Autodesk Fusion 360 part; units mm, degrees
sketch "Sketch1" plane through (0, 0, 0) normal (0, 0, 1) x (1, 0, 0)
  line L0 (-35.5, 22) -> (35.5, 22)
  line L1 (35.5, 22) -> (35.5, -22)
  line L2 (35.5, -22) -> (-35.5, -22)
  line L3 (-35.5, -22) -> (-35.5, 22)
  line L4 (0, 0) -> (-35.5, 0) construction
  line L5 (0, 0) -> (0, 22) construction
  circle A0 centre (-32.5, 19) radius 1.5
  circle A1 centre (32.5, 19) radius 1.5
  circle A2 centre (-32.5, -19) radius 1.5
  circle A3 centre (32.5, -19) radius 1.5
  point P0 (-35.5, 0)
  point P1 (0, 22)
  dimension "d1" = 71
  dimension "d2" = 44
  dimension "d3" = 3
  dimension "d4" = 3
  dimension "d5" = 3
  dimension "d8" = 65
  dimension "d9" = -38
extrude "Extrude1" add sketch "Sketch1" along normal blind 1.591
Build history of the part. All positions in model axes, mm. Coordinates: 2 decimals unless noted, no trailing zeros. Order: outer loops, then holes, each group sorted by start corner. A loop starts at its lowest first (then second) coordinate and runs counter-clockwise, first axis right, second up. Notation, with made-up numbers: (1.5, 74) - (11.5, 74) arc R18 ccw to (11.5, 98) - close; hole circle Ø5 at (74.5, -2.5). An arc over 180 degrees is marked (long way). Write each question's results on one line, items separated by ' | '. Start each with the question number.
Item 1: Band-saw the part on A-A on y = -19. Write the cut outline in (x, z), and give its area (3 significant figures).
Item 2: Band-saw the part on B-B on x = 32.5. Write the cut outline in (y, z).
Item 3: Flat gauge pins, fed straight in: pin 1 (4 mm diameter, centred on x = -32.5, y = -19, fed in from -Z); pin 2 (2.5 mm diameter, centred on x = 32.5, y = -19, fed in from -Z). Where does each tip first touch, or does it go through?
Item 4: Mould opens along X. For faces 1 (the face through (-35.5, 0, 1)), 2 (the face through (0, -22, 1)), 3 (the face through (35.5, 0, 1)), 4 (the face through (31.39, 17.99, 0.78)) say: released by +X, released by -X, zero draft, split by the parting line, or undercut.
Item 5: Wall check: probe 1 along Y at (x, z) = (32.5, 1); probe 2 along X at (y, z) = (18, 1.4). Give the ranges that are in metal, low to high. Write a range as [from, to].
Numbers:
1) outline: (-35.5, 0) - (-34, 0) - (-34, 1.59) - (-35.5, 1.59) - close; (-31, 0) - (31, 0) - (31, 1.59) - (-31, 1.59) - close; (34, 0) - (35.5, 0) - (35.5, 1.59) - (34, 1.59) - close | area: 103 mm^2
2) outline: (-22, 0) - (-20.5, 0) - (-20.5, 1.59) - (-22, 1.59) - close; (-17.5, 0) - (17.5, 0) - (17.5, 1.59) - (-17.5, 1.59) - close; (20.5, 0) - (22, 0) - (22, 1.59) - (20.5, 1.59) - close
3) pin 1: z = 0 | pin 2: through
4) face 1: released by -X | face 2: zero draft | face 3: released by +X | face 4: undercut
5) probe 1: [-22, -20.5], [-17.5, 17.5], [20.5, 22] | probe 2: [-35.5, -33.62], [-31.38, 31.38], [33.62, 35.5]
